Read the model definition and answer for the solid it produces. Units are mm, in the model's axes. Give positions to 0.01 mm unless a question says otherwise; leave off trailing zeros. Order: outer loops, then holes, each group sorted by start corner. A loop starts at its lowest first (then second) coordinate and runs counter-clockwise, first axis right, second up. Notation, with made-up numbers: (28.25, -25.5) - (41.25, -25.5) arc R18 ccw to (41.25, -20.5) - close; hole circle Ø4 at (-11.5, 43.25). An arc over 180 degrees is marked (long way). Use a Markdown table: item, result. Add a question column.
1. For a pull along X with two mould halves and no side action, classify faces 1 (the cylindrical face through (-12.83, -1.27, 0.97)), 2 (the flat face through (-14.15, 0, 0)), 3 (the cylindrical face through (-13.404, -0.434, 1.952)), 4 (the cylindrical face through (12.82, -1.27, 0.97)) as released by +X, released by -X, zero draft, split by the parting line, or undercut.
2. Consider L1, parallel to X at y = 0.7, z = 1.8; L2, parallel to X at y = 1.5, z = -1.15; L3, parallel to Z at x = -7.75, y = -0.15. Determine where each line is inside the solid, lowest interval first.
3. A cutting plane is placed at A-A on x = 6. Determine the outline of the cut face in (y, z), and give its area (3 significant figures).
Autodesk Inventor part; units mm, degrees
ref_plane "YZ Plane" through (0, 0, 0) normal (1, 0, 0) x (0, 1, 0)
ref_plane "XZ Plane" through (0, 0, 0) normal (0, 1, 0) x (-1, 0, 0)
ref_plane "XY Plane" through (0, 0, 0) normal (0, 0, 1) x (1, 0, 0)
sketch "Sketch1" plane through (0, 0, 0) normal (0, 0, 1) x (1, 0, 0)
  line L0 (-14.15, 0) -> (14.15, 0)
  line L1 (14.15, 0) -> (14.15, 1.5)
  line L2 (13.65, 2) -> (13.15, 2)
  line L3 (13.15, 2) -> (13.15, 1.6)
  line L4 (13.15, 1.6) -> (12.5, 1.6)
  line L5 (12.5, 1.6) -> (12.5, 2)
  line L6 (12.5, 2) -> (-12.5, 2)
  line L7 (-12.5, 2) -> (-12.5, 1.6)
  line L8 (-12.5, 1.6) -> (-13.15, 1.6)
  line L9 (-13.15, 1.6) -> (-13.15, 2)
  line L10 (-13.15, 2) -> (-13.65, 2)
  line L11 (-14.15, 1.5) -> (-14.15, 0)
  arc A0 (-13.65, 2) -> (-14.15, 1.5) centre (-13.65, 1.5) ccw
  arc A1 (14.15, 1.5) -> (13.65, 2) centre (13.65, 1.5) ccw
  point P0 (0, 0)
  point P1 (14.15, 2)
  point P2 (-14.15, 2)
  point P3 (0, 0)
  dimension "d0" = 25
  dimension "d1" = 0.65
  dimension "d2" = 1
  dimension "d3" = 2
  dimension "d4" = 1.6
  dimension "d5" = 1.6
  dimension "d6" = 0.5
  dimension "d7" = 1
  dimension "d8" = 0.5
revolve "Revolution1" add sketch "Sketch1" angle 360 about axis through (-14.15, 0, 0) along (1, 0, 0)
equation "\"d5\" = d4"
properties part number "Component 25 (Rocker Arm Axle)"
Output values:
| question | item | result |
|---|---|---|
| 1 | face 1 | undercut |
| 1 | face 2 | released by -X |
| 1 | face 3 | zero draft |
| 1 | face 4 | undercut |
| 2 | L1 | -13.9 to -13.15, -12.5 to 12.5, 13.15 to 13.9 |
| 2 | L2 | -13.96 to -13.15, -12.5 to 12.5, 13.15 to 13.96 |
| 2 | L3 | -1.99 to 1.99 |
| 3 | outline | circle Ø4 at (0, 0) |
| 3 | area | 12.6 mm² |
